Check sheet for the modelled part. Datum: model origin and axes. Units: mm. Face numbers are marked on the shaded views. A direction names the side the tool comes from. Round coordinates to 2 decimals unless told otherwise and drop trailing zeros. Order: outer loops, then holes, each group sorted by start corner. A loop starts at its lowest first (then second) coordinate and runs counter-clockwise, first axis right, second up. Notation, with made-up numbers: (66.25, 83.25) -> (72.25, 83.25) arc R23 ccw to (72.25, 112.25) -> close; hole circle Ø2 at (-24.5, 70.5). An arc over 180 degrees is marked (long way). Answer in a Markdown table with one row per item.
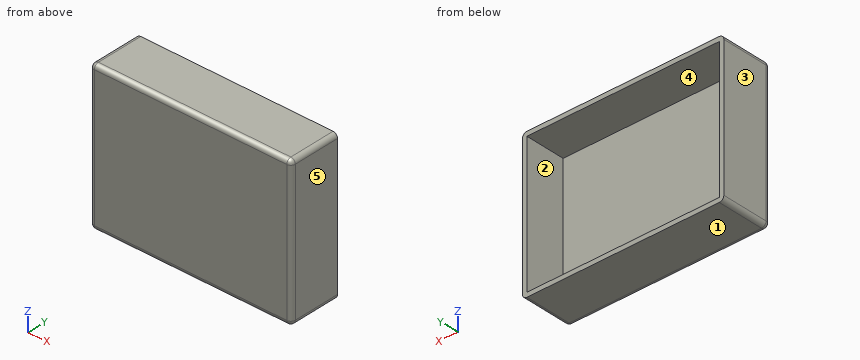
from build123d import *

# Parameters (mm, degrees)
SKETCH1_W           = 450
SKETCH1_H           = 330
BOSS_EXTRUDE1_DEPTH = 115
SKETCH2_W           = 430
SKETCH2_H           = 310
CUT_EXTRUDE1_DEPTH  = 90
FILLET1_R           = 10


with BuildPart() as part:
    # Sketch1 → Boss-Extrude1 (new body)
    with BuildSketch(Plane(origin=(0, 0, 0), x_dir=(1, 0, 0), z_dir=(0, 1, 0))):
        with Locations((162.172357903, 131.565585437)):
            Rectangle(SKETCH1_W, SKETCH1_H)
    extrude(amount=BOSS_EXTRUDE1_DEPTH)

    # Sketch2 → Cut-Extrude1 (cut)
    with BuildSketch(Plane(origin=(0, 115, 0), x_dir=(1, 0, 0), z_dir=(0, 1, 0))):
        with Locations((162.172357903, 131.565585437)):
            Rectangle(SKETCH2_W, SKETCH2_H)
    extrude(amount=-CUT_EXTRUDE1_DEPTH, mode=Mode.SUBTRACT)

    # Fillet1
    fillet1_edges = [part.edges().sort_by_distance(p)[0] for p in [
        (162.172357903, 0, -296.565585437),
        (387.172357903, 0, -131.565585437),
        (162.172357903, 0, 33.434414563),
        (-62.827642097, 0, -131.565585437),
        (-62.827642097, 57.5, -296.565585437),
        (387.172357903, 57.5, -296.565585437),
        (387.172357903, 57.5, 33.434414563),
        (-62.827642097, 57.5, 33.434414563),
    ]]
    fillet(fillet1_edges, radius=FILLET1_R)


solid = part.part
Item 1: Cross-section at C-C (z = -17). Record the boundary of the cut face in (x, y), and give its area (3 significant figures).
Result sheet:
| item | result |
|---|---|
| outline | (-62.83, 10) arc R10 ccw to (-52.83, 0) -> (377.17, 0) arc R10 ccw to (387.17, 10) -> (387.17, 115) -> (377.17, 115) -> (377.17, 25) -> (-52.83, 25) -> (-52.83, 115) -> (-62.83, 115) -> close |
| area | 13,000 mm^2 |
Item 2: Set-up check for the marked faces 4 and 5: record each of +Z, -Z, +X, -X, +Y, -Y from which the full face is reachable in a straight line by a thin tool's end or side.
Result sheet:
| item | result |
|---|---|
| face 4 | +Y |
| face 5 | +Z, -Z, +X, +Y, -Y |
Item 3: Scan lines: line 1 (X direction, y = 65.5, z = -112.5); line 2 (Z direction, x = 200, y = 97); line 3 (Y direction, x = 343, z = -4). Record each from-to range of solid material in increasing order. Write a range as [from, to].
Result sheet:
| item | result |
|---|---|
| line 1 | x = [-62.83, -52.83], [377.17, 387.17] |
| line 2 | z = [-296.57, -286.57], [23.43, 33.43] |
| line 3 | y = [0, 25] |
Item 4: Cross-section at B-B (y = 49.5). Record the boundary of the cut face in (x, z).
Result sheet:
| item | result |
|---|---|
| outline | (-62.83, -286.57) arc R10 ccw to (-52.83, -296.57) -> (377.17, -296.57) arc R10 ccw to (387.17, -286.57) -> (387.17, 23.43) arc R10 ccw to (377.17, 33.43) -> (-52.83, 33.43) arc R10 ccw to (-62.83, 23.43) -> close; hole (-52.83, -286.57) -> (377.17, -286.57) -> (377.17, 23.43) -> (-52.83, 23.43) -> close |
Item 5: Cross-section at A-A (x = -16). Record the boundary of the cut face in (y, z).
Result sheet:
| item | result |
|---|---|
| outline | (0, -286.57) arc R10 ccw to (10, -296.57) -> (115, -296.57) -> (115, -286.57) -> (25, -286.57) -> (25, 23.43) -> (115, 23.43) -> (115, 33.43) -> (10, 33.43) arc R10 ccw to (0, 23.43) -> close |
Item 6: Mould release check, pull along Z, two halves, no side actions. Record for the marked faces 1, 2 and 3: pulls with the +Z half, pulls with the -Z half, needs draft (parallel to the pull), parting line crosses it, or undercut.
Result sheet:
| item | result |
|---|---|
| face 1 | pulls with the -Z half |
| face 2 | undercut |
| face 3 | needs draft |
